Autodesk Inventor part; units mm, degrees
ref_plane "YZ Plane" through (0, 0, 0) normal (1, 0, 0) x (0, 1, 0)
ref_plane "XZ Plane" through (0, 0, 0) normal (0, 1, 0) x (-1, 0, 0)
ref_plane "XY Plane" through (0, 0, 0) normal (0, 0, 1) x (1, 0, 0)
sketch "スケッチ1" plane through (0, 0, 0) normal (1, 0, 0) x (0, 1, 0)
  line L0 (-5, 30) -> (5, 30)
  line L1 (5, 30) -> (5, 0)
  line L2 (5, 0) -> (-5, 0)
  line L3 (-5, 0) -> (-5, 30)
  line L4 (-15, 40) -> (15, 40)
  line L5 (15, 40) -> (15, 30)
  line L6 (15, 30) -> (-15, 30)
  line L7 (-15, 30) -> (-15, 40)
  line L8 (15, 30) -> (5, 0)
  line L9 (-5, 0) -> (-15, 30)
  point P0 (0, 0)
  point P1 (0, 0)
  point P2 (0, 30)
  dimension "d0" = 10
  dimension "d1" = 30
  dimension "d2" = 30
  dimension "d3" = 10
extrude "押し出し1" add sketch "スケッチ1" along normal blind 2
sketch "スケッチ2" plane through (2, 0, 0) normal (1, 0, 0) x (0, 0, -1)
  line L0 (0, -5) -> (0, 5)
  line L1 (-30, 15) -> (-40, 15)
  line L2 (-40, -15) -> (-30, -15)
  point P0 (0, 0)
  point P1 (-35, 10)
  point P2 (-35, -10)
  point P3 (-25, 0)
  point P4 (-5, 0)
  point P5 (0, 0)
  point P6 (-35, 15)
  dimension "d6" = 5
  dimension "d7" = 20
  dimension "d8" = 5
  dimension "d9" = 5
hole "穴1" at (2, 10, 35) at (2, -10, 35) at (2, 0, 25) at (2, 0, 5) direction (-1, 0, 0) diameter 3.2 end through all
properties part number "FrameJointT1515" material "アルミニウム 6061"
Design review of the part built by this model. Coordinates are the model's own, in mm. Give positions to 0.01 mm unless a question says otherwise; leave off trailing zeros. Order: outer loops, then holes, each group sorted by start corner. A loop starts at its lowest first (then second) coordinate and runs counter-clockwise, first axis right, second up. Notation, with made-up numbers: (-38.75, 64) -> (-23.75, 64) arc R25 cw to (-23.75, 86) -> close; hole circle Ø2 at (-14, -6). An arc over 180 degrees is marked (long way). Write item = value, one per line. Start each with the question number.
(1) To check wall thickness, follow line 1 along Y through (x, z) = (1.2, 35); line 2 along Z through (x, y) = (0.95, 0); line 3 along Y through (x, z) = (1.75, 24). State the ranges of each line that lie inside material, in increasing order.
(2) We need section A-A on y = -10. Write out the cut boundary in (x, z), plus the area to 3 significant figures.
(3) Mouldability with a two-part tool opening along Z and no side actions: class faces 1 (the face through (0.99, -8.44, 35.35)), 2 (the face through (1, 10, 15)), 3 (the face through (0.99, -0.07, 6.6)), 4 (the face through (2, 0, 20)) as +Z half, -Z half, draft (parallel to the pull), parting line (faces both ways), or undercut.
(4) We need section C-C on z = 5. Write out the cut boundary in (x, y).
(5) For pin 1 (1 mm diameter, centred on y = -6.5, z = 35, fed in from -X); pin 2 (1.9 mm diameter, centred on y = 0, z = 5, fed in from -X), all flat-tipped, find the tip position at first contact; note any pin that passes through.
(6) We need section B-B on x = 1.25. Write out the cut boundary in (y, z), plus the area to 3 significant figures.
(7) We need section D-D on y = -1. Write out the cut boundary in (x, z), plus the area to 3 significant figures.
Numbers:
q1.line_1 = -15 to -11.6, -8.4 to 8.4, 11.6 to 15
q1.line_2 = 0 to 3.4, 6.6 to 23.4, 26.6 to 40
q1.line_3 = -13 to -1.25, 1.25 to 13
q2.outline = (0, 15) -> (2, 15) -> (2, 33.4) -> (0, 33.4) -> close; (0, 36.6) -> (2, 36.6) -> (2, 40) -> (0, 40) -> close
q2.area = 43.6 mm^2
q3.face_1 = undercut
q3.face_2 = -Z half
q3.face_3 = undercut
q3.face_4 = draft
q4.outline = (0, -6.67) -> (2, -6.67) -> (2, -1.6) -> (0, -1.6) -> close; (0, 1.6) -> (2, 1.6) -> (2, 6.67) -> (0, 6.67) -> close
q5.pin_1 = 0
q5.pin_2 = through
q6.outline = (-15, 30) -> (-5, 0) -> (5, 0) -> (15, 30) -> (15, 40) -> (-15, 40) -> close; hole circle Ø3.2 at (-10, 35); hole circle Ø3.2 at (0, 5); hole circle Ø3.2 at (0, 25); hole circle Ø3.2 at (10, 35)
q6.area = 868 mm^2
q7.outline = (0, 0) -> (2, 0) -> (2, 3.75) -> (0, 3.75) -> close; (0, 6.25) -> (2, 6.25) -> (2, 23.75) -> (0, 23.75) -> close; (0, 26.25) -> (2, 26.25) -> (2, 40) -> (0, 40) -> close
q7.area = 70.0 mm^2
